```python
from build123d import *
from OCP.BRepFilletAPI import BRepFilletAPI_MakeChamfer

# Parameters (mm, degrees)
BOSS_EXTRUDE1_DEPTH                            = 10
BOSS_EXTRUDE2_REACH                            = 30.089
SKETCH2_R                                      = 5.5
CUT_EXTRUDE1_START                             = 20
SKETCH3_R                                      = 5.5
CUT_EXTRUDE1_DEPTH                             = 20
CSK_FOR_8_FLAT_HEAD_MACHINE_SCREW1_D           = 4.4958
CSK_FOR_8_FLAT_HEAD_MACHINE_SCREW1_CSINK_D     = 8.4328
CSK_FOR_8_FLAT_HEAD_MACHINE_SCREW1_CSINK_ANGLE = 82
CHAMFER1_SIZE                                  = 1
CHAMFER1_SIZE2                                 = 0.721110255


with BuildPart() as part:
    # Sketch1 → Boss-Extrude1 (new, symmetric)
    with BuildSketch(Plane(origin=(0, 0, 0), x_dir=(0, 0, -1), z_dir=(1, 0, 0))):
        Polygon((0, 0), (30, 0), (0, -20), align=None)
    extrude(amount=BOSS_EXTRUDE1_DEPTH, both=True)

    # Sketch2 → Boss-Extrude2 (add, up to next)
    with BuildSketch(Plane.XY.offset(-17), mode=Mode.PRIVATE) as boss_extrude2_sk1:
        with Locations((0, -10)):
            Circle(SKETCH2_R)
    boss_extrude2_tool1 = extrude(boss_extrude2_sk1.sketch, amount=BOSS_EXTRUDE2_REACH, mode=Mode.PRIVATE) - part.part
    add(boss_extrude2_tool1.solids().sort_by_distance((0, -10, -17))[0])

    # Sketch3 → Cut-Extrude1 (cut)
    with BuildSketch(Plane(origin=(0, 0, -17), x_dir=(-1, 0, 0), z_dir=(0, 0, -1)).offset(CUT_EXTRUDE1_START)):
        with Locations((0, -10)):
            Circle(SKETCH3_R)
    extrude(amount=-CUT_EXTRUDE1_DEPTH, mode=Mode.SUBTRACT)

    # CSK for #8 Flat Head Machine Screw1 (through all)
    with Locations(Plane(origin=(0, 0, -17), x_dir=(-1, 0, 0), z_dir=(0, 0, -1))):
        with Locations((0, -10)):
            CounterSinkHole(CSK_FOR_8_FLAT_HEAD_MACHINE_SCREW1_D / 2, CSK_FOR_8_FLAT_HEAD_MACHINE_SCREW1_CSINK_D / 2, counter_sink_angle=CSK_FOR_8_FLAT_HEAD_MACHINE_SCREW1_CSINK_ANGLE)

    # Chamfer1: one chamfer whose edges measure the first distance from different faces: ONE call of the kernel's chamfer builder (chamfer() names one face for all edges)
    chamfer1_edges_1 = [part.edges().sort_by_distance(p)[0] for p in [
        (-2.2479, -10, 0),
        (-10, -10, 0),
        (10, -10, 0),
        (0, 0, 0),
    ]]
    chamfer1_edges_2 = [part.edges().sort_by_distance(p)[0] for p in [
        (0, -20, 0),
    ]]
    chamfer1_side_2 = [part.faces().sort_by_distance(p)[0] for p in [
        (0, -19.717157288, 0),
    ]]
    chamfer1 = BRepFilletAPI_MakeChamfer(part.part.solid().wrapped)
    for e in chamfer1_edges_1:
        chamfer1.Add(CHAMFER1_SIZE, e.wrapped)
    for e in chamfer1_edges_2:
        chamfer1.Add(CHAMFER1_SIZE, CHAMFER1_SIZE2, e.wrapped, chamfer1_side_2[0].wrapped)  # the first distance lies on this face
    add(Compound.cast(chamfer1.Shape()), mode=Mode.REPLACE)


solid = part.part
```
Source: CAD feature listing. Evaluate the final solid. Frame: model axes, mm. A direction names the side the tool comes from. Give positions to 0.01 mm unless a question says otherwise; leave off trailing zeros. Write each loop counter-clockwise with the first axis right and the second up, starting at its lowest first coordinate (ties: lowest second). Pieces come first, ordered by that corner, then holes. Notation, with made-up numbers: (70.25, 30) - (127.25, 30) arc R30 cw to (127.25, 65) - close; hole circle Ø6 at (-17, 85.25). An arc over 180 degrees is marked (long way). One line per item, written item: value. Start each with the question number.
Q1. Section query A-A, the plane x = 0. Return the cut outline in (y, z), then the cut area to 3 significant figures.
Q2. Set-up query: faces 5 (the face through (-9.5, -9.9, -0.5)), 6 (the face through (2, -14, -17)). Return all of +Z, -Z, +X, -X, +Y, -Y with unobstructed straight access to the full face (end or side cutting, diameter ignored); none if empty.
Q3. Material intervals for probe 1 along X at (y, z) = (-10, -6.5); probe 2 along Y at (x, z) = (0, -10.5); probe 3 along Y at (x, z) = (6, -4.5), sorted ascending. Write a range as from..to.
Q4. Draft query along Y for faces 1 (the face through (0, -6, 0)), 2 (the face through (-0.29, -7.77, -7.77)), 3 (the face through (-0.51, -12.29, -14.85)), 4 (the face through (0, 0, -15)). Return one class per face: +Y half, -Y half, draft (parallel to the pull), parting line (faces both ways), or undercut.
Q5. Section query B-B, the plane y = -10. Return the cut outline in (x, z), then the cut area to 3 significant figures.
Q6. Section query C-C, the plane z = -11. Return the cut outline in (x, y).
Q7. Section query D-D, the plane y = -2. Return the cut outline in (x, z), then the cut area to 3 significant figures.
Q8. First-contact query: pin 1 Ø5 at (x, y) = (0, -10) entering from -Z; pin 2 Ø2 at (x, z) = (-1, -19) entering from +Y; pin 3 Ø9 at (x, y) = (-2.5, -8.5) entering from -Z. Flat tips, straight axial feed; report the tip coordinate or a pass-through.
Answer:
1. outline: (-19.6, -0.6) - (-15.5, -6.75) - (-15.5, -17) - (-14.22, -17) - (-12.25, -14.74) - (-12.25, -1) - (-13.25, 0) - (-19, 0) - close; (-7.75, -14.74) - (-5.78, -17) - (-4.5, -17) - (-4.5, -23.25) - (0, -30) - (0, -1) - (-1, 0) - (-6.75, 0) - (-7.75, -1) - close
1. area: 239 mm2
2. face 5: +Z, -X, +Y, -Y
2. face 6: -Z, -Y
3. probe 1: x = -10..-2.25, 2.25..10
3. probe 2: y = -15.5..-12.25, -7.75..0
3. probe 3: y = -17..0
4. face 1: draft
4. face 2: undercut
4. face 3: undercut
4. face 4: +Y half
5. outline: (-10, -15) - (-5.5, -15) - (-5.5, -17) - (-4.22, -17) - (-2.25, -14.74) - (-2.25, -1) - (-3.25, 0) - (-9, 0) - (-10, -1) - close; (2.25, -14.74) - (4.22, -17) - (5.5, -17) - (5.5, -15) - (10, -15) - (10, -1) - (9, 0) - (3.25, 0) - (2.25, -1) - close
5. area: 239 mm2
6. outline: (-10, -12.67) - (-4.81, -12.67) arc R5.5 ccw to (4.81, -12.67) - (10, -12.67) - (10, 0) - (-10, 0) - close; hole circle Ø4.5 at (0, -10)
7. outline: (-10, -27) - (10, -27) - (10, -1) - (9, 0) - (-9, 0) - (-10, -1) - close
7. area: 539 mm2
8. pin 1: stops at z = -15.03
8. pin 2: stops at y = 0
8. pin 3: stops at z = -24
